Read the model definition and answer for the solid it produces. Units are mm, in the model's axes. Face numbers are marked on the shaded views. A direction names the side the tool comes from. Give positions to 0.01 mm unless a question says otherwise; leave off trailing zeros. Order: outer loops, then holes, each group sorted by start corner. A loop starts at its lowest first (then second) coordinate and runs counter-clockwise, first axis right, second up. Notation, with made-up numbers: (75, 21.25) -> (88, 21.25) arc R11 cw to (88, 33.25) -> close; hole circle Ø9 at (87, 75.5). An arc over 180 degrees is marked (long way). Answer as CSV lines item,"result". Start each with the question number.
1) Find section C-C (z = -9.5). Determine the outline of the cut face in (x, y), and give its area (3 significant figures).
2) Straight lines are drawn through the part: L1, parallel to Z at x = 0, y = 6.5; L2, parallel to Z at x = -6, y = 3. For each, find the intervals that lie inside material, in ascending order. Write a range as from..to.
3) For the marked faces 1, 2, 3 and 4, determine the directions among +Z, -Z, +X, -X, +Y, -Y from which every point of the face is accessible in a straight line to the end or side of a thin tool.
4) Find section D-D (x = 9). Determine the outline of the cut face in (y, z).
5) Find section A-A (z = -2.5). Determine the outline of the cut face in (x, y), and give its area (3 significant figures).
6) Flat-ended cylindrical pins translate along their axes: pin 1 Ø0.6 at (y, z) = (2, -0.5) entering from -X; pin 2 Ø4 at (x, z) = (5, 5) entering from -Y; pin 3 Ø2 at (x, z) = (3.5, -2.5) entering from +Y. Find the tip coordinate at first contact, or state that the pin passes through.
7) Find section B-B (x = -8.25). Determine the outline of the cut face in (y, z), and give its area (3 significant figures).
```python
from build123d import *

# Parameters (mm, degrees)
SKETCH1_R           = 13
BOSS_EXTRUDE1_DEPTH = 6
SKETCH2_W           = 2
SKETCH2_H           = 0.4
BOSS_EXTRUDE2_DEPTH = 0.2
SKETCH3_W           = 2
SKETCH3_H           = 0.4
BOSS_EXTRUDE3_DEPTH = 0.2
SKETCH4_W           = 2
SKETCH4_H           = 0.4
BOSS_EXTRUDE4_DEPTH = 0.2
CHAMFER1_SIZE       = 0.2
SKETCH5_W           = 2
SKETCH5_H           = 0.4
BOSS_EXTRUDE5_DEPTH = 0.2
CHAMFER2_SIZE       = 0.2
SKETCH6_W           = 26
SKETCH6_H           = 26
BOSS_EXTRUDE6_DEPTH = 2
SKETCH7_R           = 11
CUT_EXTRUDE1_DEPTH  = 2
BOSS_EXTRUDE7_DEPTH = 26


with BuildPart() as part:
    # Sketch1 → Boss-Extrude1 (new body)
    with BuildSketch(Plane(origin=(0, 0, 0), x_dir=(1, 0, 0), z_dir=(0, 1, 0))):
        with Locations(Location((0, 0, 0), (0, 0, 270))):
            Circle(SKETCH1_R)
        with BuildLine():
            Line((-1, 10.95445115), (1, 10.95445115))
            ThreePointArc((1, 10.95445115), (7.778174593, 7.778174593), (10.95445115, 1))
            Line((10.95445115, 1), (10.95445115, -1))
            ThreePointArc((10.95445115, -1), (7.778174593, -7.778174593), (1, -10.95445115))
            Line((1, -10.95445115), (-1, -10.95445115))
            ThreePointArc((-1, -10.95445115), (-7.778174593, -7.778174593), (-10.95445115, -1))
            Line((-10.95445115, -1), (-10.95445115, 1))
            ThreePointArc((-10.95445115, 1), (-7.778174593, 7.778174593), (-1, 10.95445115))
        make_face(mode=Mode.SUBTRACT)
    extrude(amount=BOSS_EXTRUDE1_DEPTH)

    # Sketch2 → Boss-Extrude2 (add)
    with BuildSketch(Plane.XY.offset(-10.95445115)):
        with Locations((0, 0.2)):
            Rectangle(SKETCH2_W, SKETCH2_H)
    extrude(amount=BOSS_EXTRUDE2_DEPTH)

    # Sketch3 → Boss-Extrude3 (add)
    with BuildSketch(Plane(origin=(-10.95445115, 0, 0), x_dir=(0, 0, -1), z_dir=(1, 0, 0))):
        with Locations((0, 0.2)):
            Rectangle(SKETCH3_W, SKETCH3_H)
    extrude(amount=BOSS_EXTRUDE3_DEPTH)

    # Sketch4 → Boss-Extrude4 (add)
    with BuildSketch(Plane(origin=(0, 0, 10.95445115), x_dir=(-1, 0, 0), z_dir=(0, 0, -1))):
        with Locations((0, 0.2)):
            Rectangle(SKETCH4_W, SKETCH4_H)
    extrude(amount=BOSS_EXTRUDE4_DEPTH)

    # Chamfer1
    chamfer1_edges = [part.edges().sort_by_distance(p)[0] for p in [
        (1, 0.2, -10.75445115),
        (-1, 0.2, -10.75445115),
        (-10.75445115, 0.2, 1),
        (-10.75445115, 0.2, -1),
        (-1, 0.2, 10.75445115),
        (1, 0.2, 10.75445115),
    ]]
    chamfer(chamfer1_edges, length=CHAMFER1_SIZE - 0.0001)  # a hair under: the kernel refuses the full size

    # Sketch5 → Boss-Extrude5 (add)
    with BuildSketch(Plane.ZY.offset(-10.95445115)):
        with Locations((0, 0.2)):
            Rectangle(SKETCH5_W, SKETCH5_H)
    extrude(amount=BOSS_EXTRUDE5_DEPTH)

    # Chamfer2
    chamfer2_edges = [part.edges().sort_by_distance(p)[0] for p in [
        (10.75445115, 0.2, 1),
        (10.75445115, 0.2, -1),
    ]]
    chamfer(chamfer2_edges, length=CHAMFER2_SIZE - 0.0001)  # a hair under: the kernel refuses the full size

    # Sketch6 → Boss-Extrude6 (add)
    with BuildSketch(Plane(origin=(0, 6, 0), x_dir=(1, 0, 0), z_dir=(0, 1, 0))):
        Rectangle(SKETCH6_W, SKETCH6_H)
    extrude(amount=BOSS_EXTRUDE6_DEPTH)

    # Sketch7 → Cut-Extrude1 (cut)
    with BuildSketch(Plane.XZ.offset(-6)):
        with Locations(Location((0, 0, 0), (0, 0, 270))):
            Circle(SKETCH7_R)
    extrude(amount=-CUT_EXTRUDE1_DEPTH, mode=Mode.SUBTRACT)

    # Sketch8 → Boss-Extrude7 (add)
    with BuildSketch(Plane(origin=(13, 0, 0), x_dir=(0, 0, -1), z_dir=(1, 0, 0))):
        Polygon((-13, 8), (12.000151011, 33.000151011), (13, 32.000302023), (-11.000302023, 8), align=None)
    extrude(amount=-BOSS_EXTRUDE7_DEPTH)


solid = part.part
```
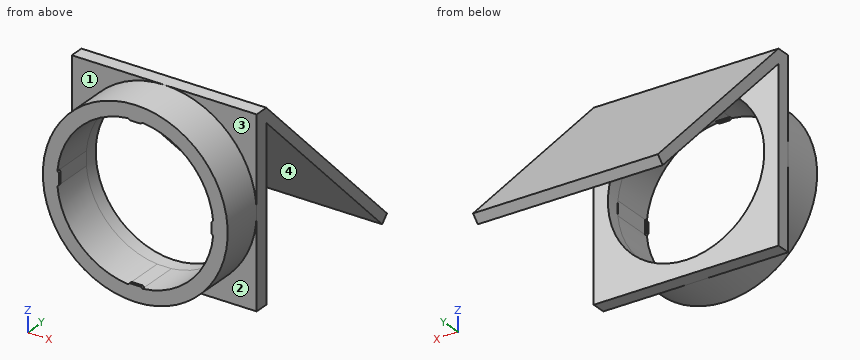
Findings below:
1,outline,"(-13, 6) -> (-8.87, 6) -> (-8.87, 0) -> (-5.55, 0) -> (-5.55, 8) -> (-13, 8) -> close; (-13, 28.5) -> (13, 28.5) -> (13, 30.5) -> (-13, 30.5) -> close; (5.55, 0) -> (8.87, 0) -> (8.87, 6) -> (13, 6) -> (13, 8) -> (5.55, 8) -> close"
1,area,"122 mm²"
2,L1,"-13..-11, 11..13"
2,L2,"-11.53..-9.22, 9.22..11.53"
3,face 1,"+Z, -X, -Y"
3,face 2,"-Z, +X, -Y"
3,face 3,"+Z, +X, -Y"
3,face 4,"-Z, +X, -X"
4,outline,"(0, -9.38) -> (6, -9.38) -> (6, -13) -> (8, -13) -> (8, -6.32) -> (0, -6.32) -> close; (0, 6.32) -> (8, 6.32) -> (8, 11) -> (32, -13) -> (33, -12) -> (8, 13) -> (6, 13) -> (6, 9.38) -> (0, 9.38) -> close"
5,outline,"(-13, 6) -> (-12.76, 6) -> (-12.76, 0) -> (-10.71, 0) -> (-10.71, 8) -> (-13, 8) -> close; (-13, 21.5) -> (13, 21.5) -> (13, 23.5) -> (-13, 23.5) -> close; (10.71, 0) -> (12.76, 0) -> (12.76, 6) -> (13, 6) -> (13, 8) -> (10.71, 8) -> close"
5,area,"85.7 mm²"
6,pin 1,"x = -13"
6,pin 2,"y = 12"
6,pin 3,"y = 24.5"
7,outline,"(0, -10.05) -> (6, -10.05) -> (6, -13) -> (8, -13) -> (8, -7.28) -> (0, -7.28) -> close; (0, 7.28) -> (8, 7.28) -> (8, 11) -> (32, -13) -> (33, -12) -> (8, 13) -> (6, 13) -> (6, 10.05) -> (0, 10.05) -> close"
7,area,"105 mm²"
